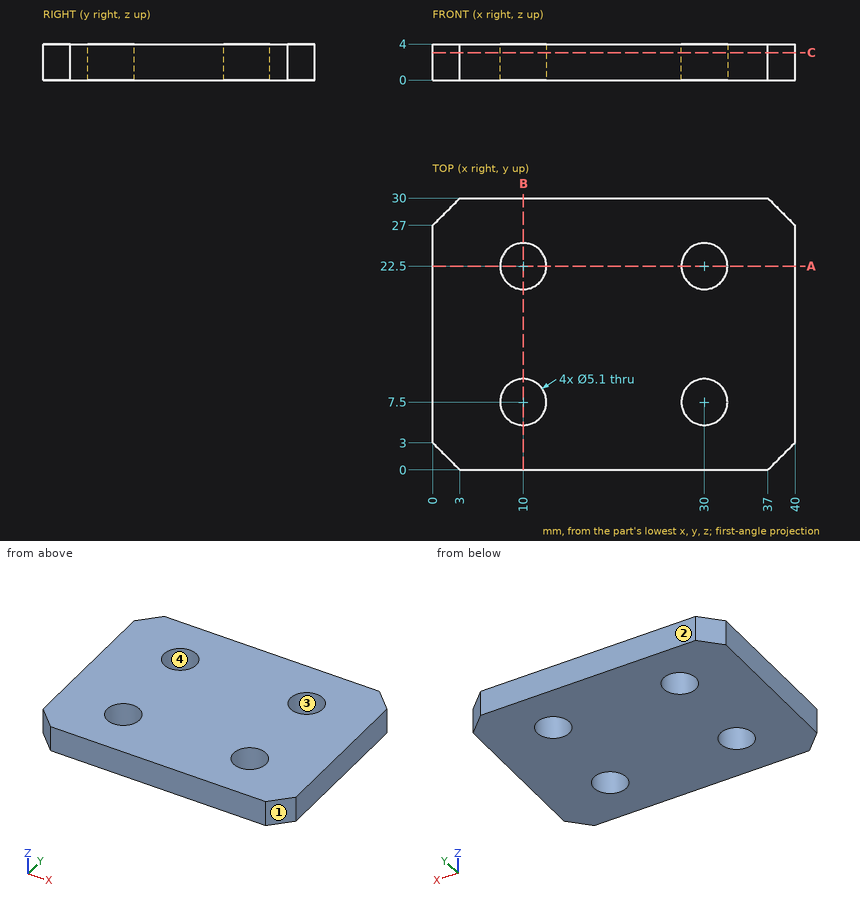
Source: three-view drawing plus pictorial views. Frame: mm from the lowest corner of the part. Round coordinates to 2 decimals unless told otherwise and drop trailing zeros. Loops run counter-clockwise (first coordinate to the right, second up) from the corner with the lowest first, then second, coordinate; pieces in that order, holes last.
1. Mould query, pull axis Y, two halves, no side actions, for the marked faces 1, 2, 3 and 4. Classes: released by +Y, released by -Y, zero draft, split by the parting line, or undercut.
2. Section query A-A on y = 22.5. Output: boundary loops of the cut face in (x, z), and give its area (3 significant figures).
3. Section query B-B on x = 10. Output: boundary loops of the cut face in (y, z), and give its area (3 significant figures).
4. Ray query, L1, parallel to Y at x = 30, z = 1.8; L2, parallel to X at y = 21, z = 1.85; L3, parallel to Y at x = 12, z = 2.45. Return the intervals inside material, ascending.
5. Section query C-C on z = 3.05. Output: boundary loops of the cut face in (x, y), and give its area (3 significant figures).
Answers below:
1. face 1: released by -Y
1. face 2: released by +Y
1. face 3: undercut
1. face 4: undercut
2. outline: (0, 0) - (7.45, 0) - (7.45, 4) - (0, 4) - close; (12.55, 0) - (27.45, 0) - (27.45, 4) - (12.55, 4) - close; (32.55, 0) - (40, 0) - (40, 4) - (32.55, 4) - close
2. area: 119 mm2
3. outline: (0, 0) - (4.95, 0) - (4.95, 4) - (0, 4) - close; (10.05, 0) - (19.95, 0) - (19.95, 4) - (10.05, 4) - close; (25.05, 0) - (30, 0) - (30, 4) - (25.05, 4) - close
3. area: 79.2 mm2
4. L1: y = 0 to 4.95, 10.05 to 19.95, 25.05 to 30
4. L2: x = 0 to 7.94, 12.06 to 27.94, 32.06 to 40
4. L3: y = 0 to 5.92, 9.08 to 20.92, 24.08 to 30
5. outline: (0, 3) - (3, 0) - (37, 0) - (40, 3) - (40, 27) - (37, 30) - (3, 30) - (0, 27) - close; hole circle Ø5.1 at (10, 7.5); hole circle Ø5.1 at (10, 22.5); hole circle Ø5.1 at (30, 7.5); hole circle Ø5.1 at (30, 22.5)
5. area: 1,100 mm2
